```python
from build123d import *

# Parameters (mm, degrees)
MAIN_DEPTH    = 12.7
SKETCH2_R     = 7.9375
AXLE_DEPTH    = 12.7
SKETCH5_W     = 12.7
SKETCH5_H     = 25.4
BARWIDE_DEPTH = 12.7
SKETCH6_R     = 2.54
SCREWS_DEPTH  = 12.7


with BuildPart() as part:
    # Sketch1 → main (new body)
    with BuildSketch(Plane(origin=(0, 0, 0), x_dir=(0, 0, -1), z_dir=(1, 0, 0))):
        with BuildLine():
            Line((0, 31.75), (50.8, 31.75))
            Line((50.8, 31.75), (184.15, -139.7))
            Line((184.15, -139.7), (196.85, -139.7))
            Line((196.85, -139.7), (196.85, -152.4))
            Line((196.85, -152.4), (209.55, -152.4))
            Line((209.55, -152.4), (209.55, -139.7))
            Line((209.55, -139.7), (311.15, -165.1))
            Line((311.15, -165.1), (184.15, -165.1))
            Line((184.15, -165.1), (50.8, -31.75))
            Line((50.8, -31.75), (0, -31.75))
            ThreePointArc((0, -31.75), (-31.75, 0), (0, 31.75))
        make_face()
    extrude(amount=MAIN_DEPTH)

    # Sketch2 → axle (cut)
    with BuildSketch(Plane(origin=(12.7, 0, 0), x_dir=(0, 0, -1), z_dir=(1, 0, 0))):
        Circle(SKETCH2_R)
    extrude(amount=-AXLE_DEPTH, mode=Mode.SUBTRACT)

    # Sketch5 → barwide (cut)
    with BuildSketch(Plane(origin=(0, 36.585769231, -47.038846154), x_dir=(-1, 0, 0), z_dir=(0, 0.6139406135149222, -0.789352217376325))):
        with Locations((-6.35, -109.029668746)):
            Rectangle(SKETCH5_W, SKETCH5_H)
    extrude(amount=-BARWIDE_DEPTH, mode=Mode.SUBTRACT)

    # Sketch6 → screws (cut)
    with BuildSketch(Plane.ZY):
        with Locations((0, 23.8125)):
            Circle(SKETCH6_R)
        with Locations((20.622229928, 11.90625)):
            Circle(SKETCH6_R)
        with Locations((20.622229928, -11.90625)):
            Circle(SKETCH6_R)
        with Locations((0, -23.8125)):
            Circle(SKETCH6_R)
        with Locations((-20.622229928, -11.90625)):
            Circle(SKETCH6_R)
        with Locations((-20.622229928, 11.90625)):
            Circle(SKETCH6_R)
    extrude(amount=-SCREWS_DEPTH, mode=Mode.SUBTRACT)


solid = part.part
```
The listing builds one solid part. Answer for the finished solid, in the listing's coordinates (mm). A direction names the side the tool comes from. Round coordinates to 2 decimals unless told otherwise and drop trailing zeros. Order: outer loops, then holes, each group sorted by start corner. A loop starts at its lowest first (then second) coordinate and runs counter-clockwise, first axis right, second up. Notation, with made-up numbers: (32, 17) -> (76, 17) arc R29 cw to (76, 53) -> close; hole circle Ø1 at (21, 12.25). An arc over 180 degrees is marked (long way). Answer as CSV lines item,"result". Start each with the question number.
(1) The part is cut by section D-D (y = -51). Determine the outline of the cut face in (x, z), then the cut area to 3 significant figures.
(2) Find the intervals of material crossed by probe 1 along Y at (x, z) = (0.5, -17); probe 2 along Z at (x, y) = (2.75, -13); probe 3 along Y at (x, z) = (11.25, -197.5), in increasing order. Write a range as from..to.
(3) Flat-ended cylindrical pins translate along their axes: pin 1 Ø4 at (x, z) = (9.5, -187.5) entering from +Y; pin 2 Ø6.5 at (x, z) = (7, -203.5) entering from +Y; pin 3 Ø1.5 at (x, z) = (10, -116) entering from +Y. Find the tip coordinate at first contact, or state that the pin passes through.
(4) The part is cut by section B-B (y = 0). Determine the outline of the cut face in (x, z).
(5) For a pull along Y with two mould halves and no side action, classify faces 6 (the face through (6, -139.7, -190)), 7 (the face through (6, -146, -209.55)), 8 (the face through (6.44, -57.13, -103.84)) as +Y half, -Y half, draft (parallel to the pull), parting line (faces both ways), or undercut.
(6) The part is cut by section A-A (x = 3.5). Count the separate pieces of the cut face and the enclosed holes in it, then the cut area to 3 significant figures.
(7) The part is cut by section C-C (z = -160). Determine the outline of the cut face in (x, y), then the cut area to 3 significant figures.
(8) A tool of negligible diameter and unlimited length cuts with its end or side. For faces 1 (the face through (6.44, -7.75, 1.72)), 2 (the face through (6.439, -63.346, -116.831)), 3 (the face through (6.439, -43.296, -101.237)), 4 (the face through (6, -31.75, -26)), 5 (the face through (6, 31.75, -25)), from which of +Z, -Z, +X, -X, +Y, -Y can it reach the whole face along a straight path? Write none if from no direction.
Evaluation:
1,outline,"(0, -99.07) -> (12.7, -99.07) -> (12.7, -70.05) -> (0, -70.05) -> close"
1,area,"369 mm²"
2,probe 1,"-31.75..31.75"
2,probe 2,"-85.61..-22.91, -18.33..18.33, 22.91..28.97"
2,probe 3,"-165.1..-152.4"
3,pin 1,"y = -139.7"
3,pin 2,"y = -152.4"
3,pin 3,"y = -63.41"
4,outline,"(0, -75.49) -> (12.7, -75.49) -> (12.7, -7.94) -> (0, -7.94) -> close; (0, 7.94) -> (12.7, 7.94) -> (12.7, 31.75) -> (0, 31.75) -> close"
5,face 6,"+Y half"
5,face 7,"draft"
5,face 8,"undercut"
6,separate pieces,"1"
6,enclosed holes,"7"
6,area,"11,900 mm²"
7,outline,"(0, -140.95) -> (12.7, -140.95) -> (12.7, -108.65) -> (0, -108.65) -> close"
7,area,"410 mm²"
8,face 1,"+X, -X"
8,face 2,"+X, -X, +Y"
8,face 3,"-Z, +X, -X"
8,face 4,"+Z, +X, -X, -Y"
8,face 5,"+Z, -Z, +X, -X, +Y"
